Check sheet for the modelled part. Datum: model origin and axes. Units: mm. Face numbers are marked on the shaded views. A direction names the side the tool comes from. Round coordinates to 2 decimals unless told otherwise and drop trailing zeros. Write each loop counter-clockwise with the first axis right and the second up, starting at its lowest first coordinate (ties: lowest second). Pieces come first, ordered by that corner, then holes.
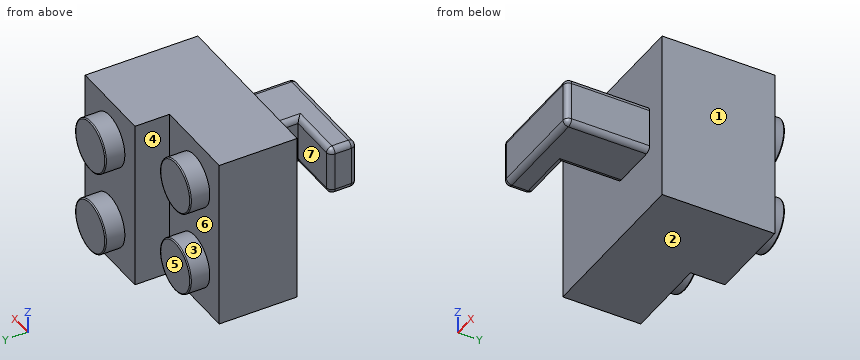
Autodesk Inventor part; units mm, degrees
ref_plane "YZ Plane" through (0, 0, 0) normal (1, 0, 0) x (0, 1, 0)
ref_plane "XZ Plane" through (0, 0, 0) normal (0, 1, 0) x (-1, 0, 0)
ref_plane "XY Plane" through (0, 0, 0) normal (0, 0, 1) x (1, 0, 0)
sketch "Sketch1" plane through (0, 0, 0) normal (0, 1, 0) x (-1, 0, 0)
  line L0 (0, 0) -> (15.8, 0)
  line L1 (15.8, 0) -> (15.8, -15.8)
  line L2 (15.8, -15.8) -> (0, -15.8)
  line L3 (0, -15.8) -> (0, 0)
  dimension "d0" = 15.8
  dimension "d1" = 15.8
extrude "Extrusion1" add sketch "Sketch1" along normal blind 3.2
sketch "Sketch2" plane through (0, 3.2, 0) normal (0, 1, 0) x (1, 0, 0)
  line L0 (-15.8, 0) -> (0, 0)
  line L1 (0, 15.8) -> (-15.8, 15.8)
  line L2 (0, 0) -> (-7.9, 0)
  line L3 (-7.9, 0) -> (-7.9, 15.8)
  line L4 (-7.9, 15.8) -> (0, 15.8)
  line L5 (0, 15.8) -> (0, 0)
  dimension "d4" = 7.9
extrude "Extrusion2" add sketch "Sketch2" along normal blind 3.2
sketch "Sketch3" plane through (0, 6.4, 0) normal (0, 1, 0) x (1, 0, 0)
  circle A0 centre (-3.9, 11.9) radius 2.4
  line L0 (0, 15.8) -> (-7.9, 15.8)
  line L1 (0, 0) -> (0, 15.8)
  line L2 (0, 7.9) -> (-7.9, 7.9) construction
  line L3 (-7.9, 15.8) -> (-7.9, 0) construction
  circle A1 centre (-3.9, 3.9) radius 2.4
  dimension "d7" = 4.8
  dimension "d8" = 3.9
  dimension "d9" = 3.9
  dimension "d10" = 8
sketch "Sketch4" plane through (0, 3.2, 0) normal (0, 1, 0) x (1, 0, 0)
  circle A0 centre (-11.9, 11.9) radius 2.4
  line L0 (-7.9, 15.8) -> (-15.8, 15.8)
  line L1 (-15.8, 15.8) -> (-15.8, 0)
  line L2 (-7.9, 15.8) -> (-7.9, 0) construction
  line L3 (-7.9, 7.9) -> (-15.8, 7.9) construction
  circle A1 centre (-11.9, 3.9) radius 2.4
  point P0 (0, 0)
  dimension "d11" = 4.8
  dimension "d12" = 3.9
  dimension "d13" = 3.9
extrude "Extrusion3" add sketch "Sketch4" along normal blind 1.8
extrude "Extrusion4" add sketch "Sketch3" along normal blind 1.8
sketch "Sketch5" plane through (0, 0, 0) normal (0, -1, 0) x (1, 0, 0)
  point P0 (0, 0)
sketch "Sketch6" plane through (0, 0, 0) normal (0, -1, 0) x (1, 0, 0)
  point P0 (0, 0)
sketch "Sketch7" plane through (0, 0, 0) normal (0, -1, 0) x (1, 0, 0)
  line L0 (-7.9, 0) -> (0, 0)
  line L1 (0, 0) -> (-15.8, 0)
  line L2 (-15.8, 0) -> (-15.8, -15.8)
  line L3 (-15.8, -15.8) -> (0, -15.8)
  line L4 (0, -15.8) -> (0, 0)
extrude "Extrusion5" add sketch "Sketch7" along normal blind 4
sketch "Sketch8" plane through (0, -4, 0) normal (0, -1, 0) x (1, 0, 0)
  line L0 (-2, -5.65) -> (-7, -5.65)
  line L1 (-7, -5.65) -> (-7, -10.15)
  line L2 (-7, -10.15) -> (-2, -10.15)
  line L3 (-2, -10.15) -> (-2, -5.65)
  line L4 (0, 0) -> (0, -15.8) construction
  line L5 (0, -7.9) -> (-15.8, -7.9) construction
  line L6 (-15.8, -15.8) -> (-15.8, 0) construction
  point P0 (-2, -7.9)
  dimension "d20" = 4.5
  dimension "d21" = 5
  dimension "d22" = 0
  dimension "d24" = 7
extrude "Extrusion6" add sketch "Sketch8" along normal blind 7.7
sketch "Sketch9" plane through (-7, -4, -10.15) normal (-1, 0, 0) x (0, 0, 1)
  point P0 (10.15, 4)
sketch "Sketch10" plane through (-7, -4, -10.15) normal (-1, 0, 0) x (0, 0, 1)
  line L0 (4.5, 0) -> (4.5, -7.7)
  line L1 (0, 0) -> (0, -7.7)
  line L2 (4.5, -7.7) -> (0, -7.7)
  line L3 (0, -7.7) -> (0, -5.2)
  line L4 (0, -5.2) -> (4.5, -5.2)
  line L5 (4.5, -5.2) -> (4.5, -7.7)
  point P0 (10.15, 4)
  point P1 (0, -7.7)
  point P2 (4.5, -5.2)
  dimension "d27" = 2.5
extrude "Extrusion7" add sketch "Sketch10" along normal blind 5
fillet "Fillet1" radius 0.1 4 edges at (-6.3, 8.2, -3.9) (-14.3, 5, -3.9) (-14.3, 5, -11.9) (-6.3, 8.2, -11.9)
fillet "Fillet2" radius 0.5 13 edges at (-2, -7.85, -5.65) (-2, -7.85, -10.15) (-7, -11.7, -5.65) (-7, -11.7, -10.15) (-12, -11.7, -7.9) (-12, -10.45, -10.15) (-12, -10.45, -5.65) (-12, -9.2, -7.9) (-9.5, -9.2, -5.65) (-9.5, -9.2, -10.15) (-7, -6.6, -10.15) (-7, -6.6, -5.65) (-2, -11.7, -7.9)
properties part number "LEGO_hanging_brick"
1. Release check for a two-part mould opening along X. For the marked faces 1, 2, 3 and 4 record: released by +X, released by -X, zero draft, split by the parting line, or undercut.
2. Sectioned sample at B-B, the plane z = -3.9. Enter the section's corners in (x, y).
3. Set-up check for the marked faces 5, 6 and 7: record each of +Z, -Z, +X, -X, +Y, -Y from which the full face is reachable in a straight line by a thin tool's end or side.
4. Sectioned sample at D-D, the plane y = 6.75. Enter the section's corners in (x, z).
5. Go/stop test with flat-tipped pins: pin 1 (1 mm diameter, centred on y = 5, z = -7, fed in from -X); pin 2 (1.8 mm diameter, centred on y = -8, z = -7.5, fed in from +X); pin 3 (1 mm diameter, centred on x = -9, z = -7.5, fed in from +Y). Record where each tip stops, or that it passes through.
6. Scan lines: line 1 along Y through (x, z) = (-11, -6.25); line 2 along Y through (x, z) = (-6.75, -3); line 3 along Y through (x, z) = (-13, -11). Record each from-to range of solid material in increasing order.
7. Sectioned sample at C-C, the plane x = -3.9. Enter the section's corners in (y, z).
8. Sectioned sample at A-A, the plane y = -5.75. Enter the section's corners in (x, z).
Computed values:
1. face 1: released by +X
1. face 2: zero draft
1. face 3: undercut
1. face 4: undercut
2. outline: (-15.8, -4) - (0, -4) - (0, 6.4) - (-1.5, 6.4) - (-1.5, 8.1) arc R0.1 ccw to (-1.6, 8.2) - (-6.2, 8.2) arc R0.1 ccw to (-6.3, 8.1) - (-6.3, 6.4) - (-7.9, 6.4) - (-7.9, 3.2) - (-9.5, 3.2) - (-9.5, 4.9) arc R0.1 ccw to (-9.6, 5) - (-14.2, 5) arc R0.1 ccw to (-14.3, 4.9) - (-14.3, 3.2) - (-15.8, 3.2) - close
3. face 5: +Z, -Z, -X, +Y
3. face 6: +Y
3. face 7: +Z, -Z, -X
4. outline: circle Ø4.8 at (-3.9, -11.9); circle Ø4.8 at (-3.9, -3.9)
5. pin 1: stops at x = -7.9
5. pin 2: stops at x = -2
5. pin 3: stops at y = 3.2
6. line 1: y = -11.7 to -9.2, -4 to 3.2
6. line 2: y = -4 to 6.4
6. line 3: y = -4 to 5
7. outline: (-11.7, -9.65) arc R0.5 ccw to (-11.2, -10.15) - (-4, -10.15) - (-4, -15.8) - (6.4, -15.8) - (6.4, -14.3) - (8.1, -14.3) arc R0.1 ccw to (8.2, -14.2) - (8.2, -9.6) arc R0.1 ccw to (8.1, -9.5) - (6.4, -9.5) - (6.4, -6.3) - (8.1, -6.3) arc R0.1 ccw to (8.2, -6.2) - (8.2, -1.6) arc R0.1 ccw to (8.1, -1.5) - (6.4, -1.5) - (6.4, 0) - (-4, 0) - (-4, -5.65) - (-11.2, -5.65) arc R0.5 ccw to (-11.7, -6.15) - close
8. outline: (-7, -9.65) arc R0.5 ccw to (-6.5, -10.15) - (-2.5, -10.15) arc R0.5 ccw to (-2, -9.65) - (-2, -6.15) arc R0.5 ccw to (-2.5, -5.65) - (-6.5, -5.65) arc R0.5 ccw to (-7, -6.15) - close
